Model file for the job. Use its own axes, mm. Face numbers are marked on the shaded views. A direction names the side the tool comes from. Give positions to 0.01 mm unless a question says otherwise; leave off trailing zeros. Write each loop counter-clockwise with the first axis right and the second up, starting at its lowest first coordinate (ties: lowest second). Pieces come first, ordered by that corner, then holes. Notation, with made-up numbers: (14.25, -17) - (19.25, -17) arc R25 ccw to (19.25, 9) - close; hole circle Ø1 at (80.25, 77.25). An arc over 180 degrees is marked (long way). One line per item, written item: value. Start each with the question number.
(1) Drop flat-ended pins along their axis: P1, Ø11.5, axis at x = 9, y = 7.5, coming from the +Z side; P2, Ø5.5, axis at y = -20.5, z = 28, coming from the -X side; P3, Ø12.5, axis at x = 0, y = 10, coming from the -Z side; P4, Ø10, axis at x = 0, y = 7, coming from the +Z side. Give the stop position or say it passes through.
(2) Probe L1, parallel to Y at x = 0, z = -2.5 (3 decimals); L2, parallel to X at y = -25.45, z = 45.6; L3, parallel to Y at x = 0, z = 0.9 (3 decimals). List the from-to ranges inside material, lowest first.
(3) Cut at D-D, the plane y = 3. List the corners of the cut face in (x, z), and give its area (3 significant figures).
(4) Cut at C-C, the plane z = 7.5. List the corners of the cut face in (x, y), and give its area (3 significant figures).
(5) Cut at B-B, the plane z = 34. List the corners of the cut face in (x, y), and give its area (3 significant figures).
(6) 3-axis set-ups, long thin cutter, end or side, ignore diameter. For the marked faces 1, 2, 3 and 4: which of +Z, -Z, +X, -X, +Y, -Y reach the whole face in a straight line?
(7) Mould opens along X. For the marked faces 5, 6 and 7 say: pulls with the +X half, pulls with the -X half, needs draft (parallel to the pull), parting line crosses it, or undercut.
(8) Cut at A-A, the plane x = -30.5. List the corners of the cut face in (y, z).
from build123d import *

# Parameters (mm, degrees)
CROQUIS1_R                 = 21.1
SALIENTE_EXTRUIR1_DEPTH    = 51.6
CROQUIS2_R                 = 18.75
CORTAR_EXTRUIR1_DEPTH      = 48.6
CROQUIS5_R                 = 7.775
CROQUIS5_R_2               = 6.275
SALIENTE_EXTRUIR3_DEPTH    = 6
CORTAR_EXTRUIR2_START      = -66
CROQUIS6_R                 = 6.275
CORTAR_EXTRUIR2_DEPTH      = 66
CROQUIS10_R                = 25
CROQUIS10_R_2              = 21.1
SALIENTE_EXTRUIR4_DEPTH    = 51.6
CROQUIS11_R                = 17.5
CROQUIS11_R_2              = 16
SALIENTE_EXTRUIR5_DEPTH    = 9
SALIENTE_EXTRUIR6_START    = -3
CROQUIS12_R                = 19
CROQUIS12_R_2              = 17.5
SALIENTE_EXTRUIR6_DEPTH    = 3
SALIENTE_EXTRUIR7_DEPTH    = 51.6
SALIENTE_EXTRUIR8_REACH    = 78.981
CROQUIS14_W                = 51.6
CROQUIS14_H                = 3
CROQUIS16_W                = 12
CROQUIS16_H                = 3
SALIENTE_EXTRUIR9_DEPTH    = 12
SALIENTE_EXTRUIR11_DEPTH   = 3
CROQUIS19_R                = 2.5
CORTAR_EXTRUIR5_DEPTH      = 15
CROQUIS20_W                = 12
CROQUIS20_H                = 3
SALIENTE_EXTRUIR12_DEPTH   = 12
SALIENTE_EXTRUIR13_DEPTH   = 3
CROQUIS22_R                = 2.5
CORTAR_EXTRUIR6_DEPTH      = 12
SALIENTE_EXTRUIR14_DEPTH   = 8
SALIENTE_EXTRUIR14_2_DEPTH = 8
CROQUIS26_W                = 2.5
CROQUIS26_H                = 8
CORTAR_EXTRUIR11_DEPTH     = 10
CROQUIS27_W                = 8
CROQUIS27_H                = 2.5
CORTAR_EXTRUIR12_DEPTH     = 13


with BuildPart() as part:
    # Croquis1 → Saliente-Extruir1 (new body)
    with BuildSketch(Plane.XY):
        with Locations(Location((0, 0, 0), (0, 0, 180))):
            Circle(CROQUIS1_R)
    extrude(amount=SALIENTE_EXTRUIR1_DEPTH)

    # Croquis2 → Cortar-Extruir1 (cut)
    with BuildSketch(Plane.XY.offset(51.6)):
        Circle(CROQUIS2_R)
    extrude(amount=-CORTAR_EXTRUIR1_DEPTH, mode=Mode.SUBTRACT)

    # Croquis5 → Saliente-Extruir3 (add)
    with BuildSketch(Plane.XY.offset(3)):
        with Locations((0, 7)):
            Circle(CROQUIS5_R)
        with Locations((0, 7)):
            Circle(CROQUIS5_R_2, mode=Mode.SUBTRACT)
    extrude(amount=-SALIENTE_EXTRUIR3_DEPTH)

    # Croquis6 → Cortar-Extruir2 (cut)
    with BuildSketch(Plane(origin=(0, 0, 0), x_dir=(-1, 0, 0), z_dir=(0, 0, -1)).offset(CORTAR_EXTRUIR2_START)):
        with Locations(Location((0, 7, 0), (0, 0, 180))):
            Circle(CROQUIS6_R)
    extrude(amount=CORTAR_EXTRUIR2_DEPTH, mode=Mode.SUBTRACT)

    # Croquis10 → Saliente-Extruir4 (add)
    with BuildSketch(Plane(origin=(0, 0, 0), x_dir=(-1, 0, 0), z_dir=(0, 0, -1))):
        Circle(CROQUIS10_R)
        Circle(CROQUIS10_R_2, mode=Mode.SUBTRACT)
    extrude(amount=-SALIENTE_EXTRUIR4_DEPTH)

    # Croquis11 → Saliente-Extruir5 (add)
    with BuildSketch(Plane(origin=(0, 0, 0), x_dir=(-1, 0, 0), z_dir=(0, 0, -1))):
        with Locations(Location((0, 7, 0), (0, 0, 180))):
            Circle(CROQUIS11_R)
        with Locations((0, 7)):
            Circle(CROQUIS11_R_2, mode=Mode.SUBTRACT)
    extrude(amount=SALIENTE_EXTRUIR5_DEPTH)

    # Croquis12 → Saliente-Extruir6 (add)
    with BuildSketch(Plane(origin=(0, 0, -9), x_dir=(-1, 0, 0), z_dir=(0, 0, -1)).offset(SALIENTE_EXTRUIR6_START)):
        with Locations((0, 7)):
            Circle(CROQUIS12_R)
        with Locations(Location((0, 7, 0), (0, 0, 180))):
            Circle(CROQUIS12_R_2, mode=Mode.SUBTRACT)
    extrude(amount=SALIENTE_EXTRUIR6_DEPTH)

    # Croquis13 → Saliente-Extruir7 (add)
    with BuildSketch(Plane(origin=(0, 0, 0), x_dir=(-1, 0, 0), z_dir=(0, 0, -1))):
        with BuildLine():
            Line((-20.673776338, -25), (0, -25))
            ThreePointArc((0, -25), (-11.695700136, -22.095488189), (-20.673776338, -14.056847866))
            Line((-20.673776338, -14.056847866), (-20.673776338, -25))
        make_face()
        with BuildLine():
            ThreePointArc((20.673776338, -14.056847866), (11.695700136, -22.095488189), (0, -25))
            Line((0, -25), (20.673776338, -25))
            Line((20.673776338, -25), (20.673776338, -14.056847866))
        make_face()
        Polygon((25, -27.632757418), (25, -25), (0, -25), (-25, -25), (-25, -27.632757418), align=None)
    extrude(amount=-SALIENTE_EXTRUIR7_DEPTH)

    # Saliente-Extruir8: up to this face of the body (flat: up to its plane)
    saliente_extruir8_end = Plane(part.part.faces().sort_by_distance((-25, -26.316378709, 25.8))[0])
    # Croquis14 → Saliente-Extruir8 (add, up to the picked face)
    with BuildSketch(Plane(origin=(25, 0, 0), x_dir=(0, 0, -1), z_dir=(1, 0, 0)), mode=Mode.PRIVATE) as saliente_extruir8_sk1:
        with Locations((-25.8, -26.132757418)):
            Rectangle(CROQUIS14_W, CROQUIS14_H)
    saliente_extruir8_tool1 = split(extrude(saliente_extruir8_sk1.sketch, amount=-SALIENTE_EXTRUIR8_REACH, mode=Mode.PRIVATE), bisect_by=saliente_extruir8_end, keep=Keep.BOTH, mode=Mode.PRIVATE)
    add(saliente_extruir8_tool1.solids().sort_by(Axis((25, -26.132757, 25.8), (-1, 0, 0)))[0])

    # Croquis16 → Saliente-Extruir9 (add)
    with BuildSketch(Plane(origin=(25, 0, 0), x_dir=(0, 0, -1), z_dir=(1, 0, 0))):
        with Locations((-45.6, -26.132757418)):
            Rectangle(CROQUIS16_W, CROQUIS16_H)
        with Locations((-6, -26.132757418)):
            Rectangle(CROQUIS16_W, CROQUIS16_H)
    extrude(amount=SALIENTE_EXTRUIR9_DEPTH)

    # Croquis18 → Saliente-Extruir11 (add)
    with BuildSketch(Plane(origin=(0, -24.632757418, 0), x_dir=(1, 0, 0), z_dir=(0, 1, 0))):
        with BuildLine():
            ThreePointArc((37, -12), (41.242640687, -10.242640687), (43, -6))
            ThreePointArc((43, -6), (41.242640687, -1.757359313), (37, 0))
            Line((37, 0), (37, -12))
        make_face()
        with BuildLine():
            Line((37, -12), (37, 0))
            ThreePointArc((37, 0), (31, -6), (37, -12))
        make_face()
        with BuildLine():
            ThreePointArc((43, -45.6), (41.242640687, -41.357359313), (37, -39.6))
            Line((37, -39.6), (37, -51.6))
            ThreePointArc((37, -51.6), (41.242640687, -49.842640687), (43, -45.6))
        make_face()
        with BuildLine():
            Line((37, -51.6), (37, -39.6))
            ThreePointArc((37, -39.6), (31, -45.6), (37, -51.6))
        make_face()
    extrude(amount=-SALIENTE_EXTRUIR11_DEPTH)

    # Croquis19 → Cortar-Extruir5 (cut)
    with BuildSketch(Plane(origin=(0, -24.632757418, 0), x_dir=(1, 0, 0), z_dir=(0, 1, 0))):
        with Locations(Location((37, -6, 0), (0, 0, 270))):
            Circle(CROQUIS19_R)
        with Locations(Location((37, -45.6, 0), (0, 0, 270))):
            Circle(CROQUIS19_R)
    extrude(amount=-CORTAR_EXTRUIR5_DEPTH, mode=Mode.SUBTRACT)

    # Croquis20 → Saliente-Extruir12 (add)
    with BuildSketch(Plane.ZY.offset(25)):
        with Locations((6, -26.132757418)):
            Rectangle(CROQUIS20_W, CROQUIS20_H)
        with Locations((45.6, -26.132757418)):
            Rectangle(CROQUIS20_W, CROQUIS20_H)
    extrude(amount=SALIENTE_EXTRUIR12_DEPTH)

    # Croquis21 → Saliente-Extruir13 (add)
    with BuildSketch(Plane(origin=(0, -24.632757418, 0), x_dir=(1, 0, 0), z_dir=(0, 1, 0))):
        with BuildLine():
            ThreePointArc((-31, -6), (-32.757359313, -1.757359313), (-37, 0))
            Line((-37, 0), (-37, -12))
            ThreePointArc((-37, -12), (-32.757359313, -10.242640687), (-31, -6))
        make_face()
        with BuildLine():
            Line((-37, -12), (-37, 0))
            ThreePointArc((-37, 0), (-43, -6), (-37, -12))
        make_face()
        with BuildLine():
            ThreePointArc((-31, -45.6), (-32.757359313, -41.357359313), (-37, -39.6))
            Line((-37, -39.6), (-37, -51.6))
            ThreePointArc((-37, -51.6), (-32.757359313, -49.842640687), (-31, -45.6))
        make_face()
        with BuildLine():
            Line((-37, -51.6), (-37, -39.6))
            ThreePointArc((-37, -39.6), (-43, -45.6), (-37, -51.6))
        make_face()
    extrude(amount=-SALIENTE_EXTRUIR13_DEPTH)

    # Croquis22 → Cortar-Extruir6 (cut)
    with BuildSketch(Plane(origin=(0, -24.632757418, 0), x_dir=(1, 0, 0), z_dir=(0, 1, 0))):
        with Locations(Location((-37, -6, 0), (0, 0, 270))):
            Circle(CROQUIS22_R)
        with Locations(Location((-37, -45.6, 0), (0, 0, 270))):
            Circle(CROQUIS22_R)
    extrude(amount=-CORTAR_EXTRUIR6_DEPTH, mode=Mode.SUBTRACT)


with BuildPart() as body_2:
    # Croquis23 → Saliente-Extruir14 (new body)
    with BuildSketch(Plane(origin=(0, 0, -9), x_dir=(-1, 0, 0), z_dir=(0, 0, -1))):
        Polygon((2.5, 29.282754404), (2.5, 26), (0, 26), (-2.5, 26), (-2.5, 29.282754404), align=None)
    extrude(amount=-SALIENTE_EXTRUIR14_DEPTH)


with BuildPart() as body_3:
    # Croquis23 → Saliente-Extruir14 2 (new body)
    with BuildSketch(Plane(origin=(0, 0, -9), x_dir=(-1, 0, 0), z_dir=(0, 0, -1))):
        Polygon((-23.376501852, 9.5), (-23.376501852, 4.5), (-19, 4.5), (-19, 7), (-19, 9.5), align=None)
    extrude(amount=-SALIENTE_EXTRUIR14_2_DEPTH)


with BuildPart() as cortar_extruir11_tool:
    # Croquis26 → Cortar-Extruir11 (new body)
    with BuildSketch(Plane(origin=(0, 29.282754404, 0), x_dir=(1, 0, 0), z_dir=(0, 1, 0))):
        with BuildLine():
            ThreePointArc((2.5, 9), (0, 11.5), (-2.5, 9))
            Line((-2.5, 9), (2.5, 9))
        make_face()
        with Locations((-1.25, 5)):
            Rectangle(CROQUIS26_W, CROQUIS26_H)
        with Locations((1.25, 5)):
            Rectangle(CROQUIS26_W, CROQUIS26_H)
        with BuildLine():
            Line((2.5, 1), (0, 1))
            Line((0, 1), (-2.5, 1))
            ThreePointArc((-2.5, 1), (-2.447265782, 0.489225891), (-2.291287847, 0))
            Line((-2.291287847, 0), (2.291287847, 0))
            ThreePointArc((2.291287847, 0), (2.447265782, 0.489225891), (2.5, 1))
        make_face()
    extrude(amount=-CORTAR_EXTRUIR11_DEPTH)


with BuildPart() as part_1:
    add(part.part)

    # Cortar-Extruir11: cut by cortar_extruir11_tool
    add(cortar_extruir11_tool.part, mode=Mode.SUBTRACT)


with BuildPart() as body_2_1:
    add(body_2.part)

    # Cortar-Extruir11: cut by cortar_extruir11_tool
    add(cortar_extruir11_tool.part, mode=Mode.SUBTRACT)


with BuildPart() as cortar_extruir12_tool:
    # Croquis27 → Cortar-Extruir12 (new body)
    with BuildSketch(Plane(origin=(23.376501852, 0, 0), x_dir=(0, 0, -1), z_dir=(1, 0, 0))):
        with BuildLine():
            Line((1, 4.5), (1, 7))
            Line((1, 7), (1, 9.5))
            ThreePointArc((1, 9.5), (0.489225891, 9.447265782), (0, 9.291287847))
            Line((0, 9.291287847), (0, 4.708712153))
            ThreePointArc((0, 4.708712153), (0.489225891, 4.552734218), (1, 4.5))
        make_face()
        with Locations((5, 8.25)):
            Rectangle(CROQUIS27_W, CROQUIS27_H)
        with Locations((5, 5.75)):
            Rectangle(CROQUIS27_W, CROQUIS27_H)
        with BuildLine():
            ThreePointArc((9, 4.5), (11.5, 7), (9, 9.5))
            Line((9, 9.5), (9, 4.5))
        make_face()
    extrude(amount=-CORTAR_EXTRUIR12_DEPTH)


with BuildPart() as part_2:
    add(part_1.part)

    # Cortar-Extruir12: cut by cortar_extruir12_tool
    add(cortar_extruir12_tool.part, mode=Mode.SUBTRACT)


with BuildPart() as body_3_1:
    add(body_3.part)

    # Cortar-Extruir12: cut by cortar_extruir12_tool
    add(cortar_extruir12_tool.part, mode=Mode.SUBTRACT)


solid = part_2.part
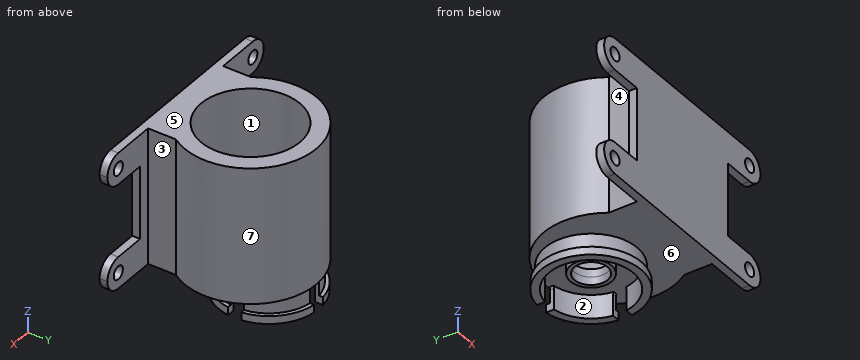
Answers follow:
1. P1: stops at z = 3
1. P2: stops at x = -20.67
1. P3: stops at z = -3
1. P4: passes through
2. L1: y = -10.5 to -9, -0.775 to 0.725, 13.275 to 14.775
2. L2: x = -43 to -39.5, -34.5 to 34.5, 39.5 to 43
2. L3: y = -27.633 to 0.725, 13.275 to 25
3. outline: (-24.82, 0) - (-17.04, 0) - (-17.04, -6) - (-18.57, -6) - (-18.57, -9) - (-15.49, -9) - (-15.49, 0) - (-6.67, 0) - (-6.67, -3) - (-4.83, -3) - (-4.83, 3) - (-18.51, 3) - (-18.51, 51.6) - (-24.82, 51.6) - close; (4.83, -3) - (6.67, -3) - (6.67, 0) - (15.49, 0) - (15.49, -9) - (18.57, -9) - (18.57, -6) - (17.04, -6) - (17.04, 0) - (24.82, 0) - (24.82, 51.6) - (18.51, 51.6) - (18.51, 3) - (4.83, 3) - close
3. area: 781 mm²
4. outline: (-42.81, -27.63) - (-39, -27.63) - (-39, -24.63) - (-42.81, -24.63) - close; (-35, -27.63) - (35, -27.63) - (35, -24.63) - (20.67, -24.63) - (20.67, -14.06) arc R25 ccw (long way) to (-20.67, -14.06) - (-20.67, -24.63) - (-35, -24.63) - close; (39, -27.63) - (42.81, -27.63) - (42.81, -24.63) - (39, -24.63) - close; hole circle Ø37.5 at (0, 0)
4. area: 1,210 mm²
5. outline: (-25, -27.63) - (25, -27.63) - (25, -24.63) - (20.67, -24.63) - (20.67, -14.06) arc R25 ccw (long way) to (-20.67, -14.06) - (-20.67, -24.63) - (-25, -24.63) - close; hole circle Ø37.5 at (0, 0)
5. area: 1,130 mm²
6. face 1: +Z
6. face 2: -Z
6. face 3: +Z, -Z, +X
6. face 4: +Z, -Z, -X
7. face 5: needs draft
7. face 6: undercut
7. face 7: parting line crosses it
8. outline: (-27.63, 0) - (-24.63, 0) - (-24.63, 12) - (-27.63, 12) - close; (-27.63, 39.6) - (-24.63, 39.6) - (-24.63, 51.6) - (-27.63, 51.6) - close
